Drawing for the job (mm, zero at the part's lowest x, y, z). A direction names the side the tool comes from. Give positions to 0.01 mm unless a question says otherwise; leave off trailing zeros. Loops run counter-clockwise (first coordinate to the right, second up) from the corner with the lowest first, then second, coordinate; pieces in that order, holes last. Notation, with made-up numbers: (31, 85) - (78, 85) arc R11 ccw to (78, 103) - close; hole circle Ø5 at (38, 40.5). An arc over 180 degrees is marked (long way). Return JSON: item names as keys, results as strings. Group by question number.
1) Drop flat-ended pins along their axis: pin 1 (8 mm diameter, centred on x = 23, y = 35.5, fed in from -Z); pin 2 (1.5 mm diameter, centred on x = 5.5, z = 7, fed in from -Y); pin 3 (2 mm diameter, centred on x = 16.5, z = 5, fed in from +Y); pin 4 (3 mm diameter, centred on x = 31, z = 17.5, fed in from +Y). Give the stop position or say it passes through.
2) Slice it at C-C (x = 26). List the corners of the cut face in (y, z).
3) Slice it at B-B (y = 26). List the corners of the cut face in (x, z).
4) Slice it at A-A (z = 12.75). List the corners of the cut face in (x, y).
5) Mould opens along X. For the marked faces 1, 2 and 3 say: released by +X, released by -X, zero draft, split by the parting line, or undercut.
6) Slice it at D-D (x = 36.5). List the corners of the cut face in (y, z) (1 decimal), and give its area (3 significant figures).
7) 3-axis set-ups, long thin cutter, end or side, ignore diameter. For the marked faces 4 and 5: which of +Z, -Z, +X, -X, +Y, -Y reach the whole face in a straight line?
8) Drill centre lines: probe 1 along Z at (x, y) = (40.5, 27); probe 2 along Y at (x, z) = (36, 6.5) (1 decimal); probe 3 along Y at (x, z) = (39.5, 2.25). Where is each one in solid material? Low to high. Write a range as from..to.
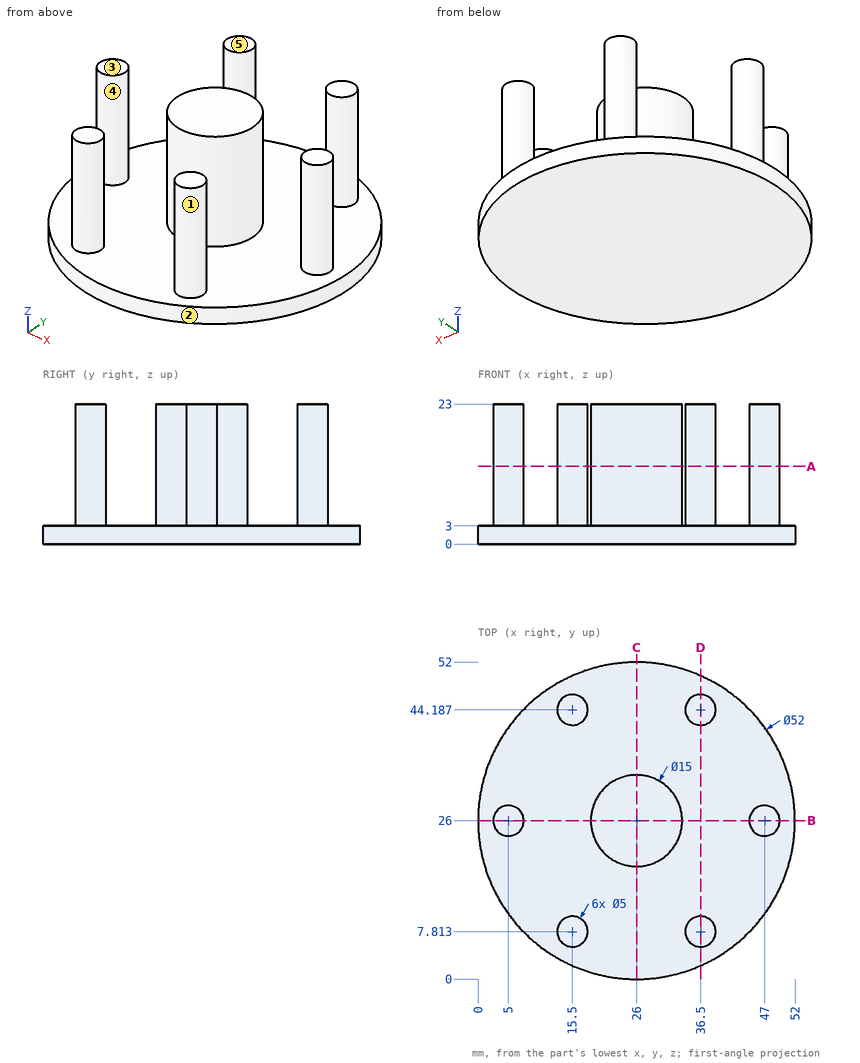
Results:
{
 "1": {"pin 1": "z = 0", "pin 2": "y = 23.5", "pin 3": "y = 46.69", "pin 4": "y = 32.63"},
 "2": {"outline": "(0, 0) - (52, 0) - (52, 3) - (33.5, 3) - (33.5, 23) - (18.5, 23) - (18.5, 3) - (0, 3) - close"},
 "3": {"outline": "(0, 0) - (52, 0) - (52, 3) - (49.5, 3) - (49.5, 23) - (44.5, 23) - (44.5, 3) - (33.5, 3) - (33.5, 23) - (18.5, 23) - (18.5, 3) - (7.5, 3) - (7.5, 23) - (2.5, 23) - (2.5, 3) - (0, 3) - close"},
 "4": {"outline": "circle Ø5 at (5, 26); circle Ø5 at (15.5, 7.81); circle Ø5 at (15.5, 44.19); circle Ø15 at (26, 26); circle Ø5 at (36.5, 7.81); circle Ø5 at (36.5, 44.19); circle Ø5 at (47, 26)"},
 "5": {"face 1": "undercut", "face 2": "split by the parting line", "face 3": "zero draft"},
 "6": {"outline": "(2.2, 0) - (49.8, 0) - (49.8, 3) - (46.7, 3) - (46.7, 23) - (41.7, 23) - (41.7, 3) - (10.3, 3) - (10.3, 23) - (5.3, 23) - (5.3, 3) - (2.2, 3) - close", "area": "343 mm2"},
 "7": {"face 4": "+Z", "face 5": "+Z, +X, -X, +Y, -Y"},
 "8": {"probe 1": "0..3", "probe 2": "5.4..10.3, 41.7..46.6", "probe 3": "3.78..48.22"}
}
